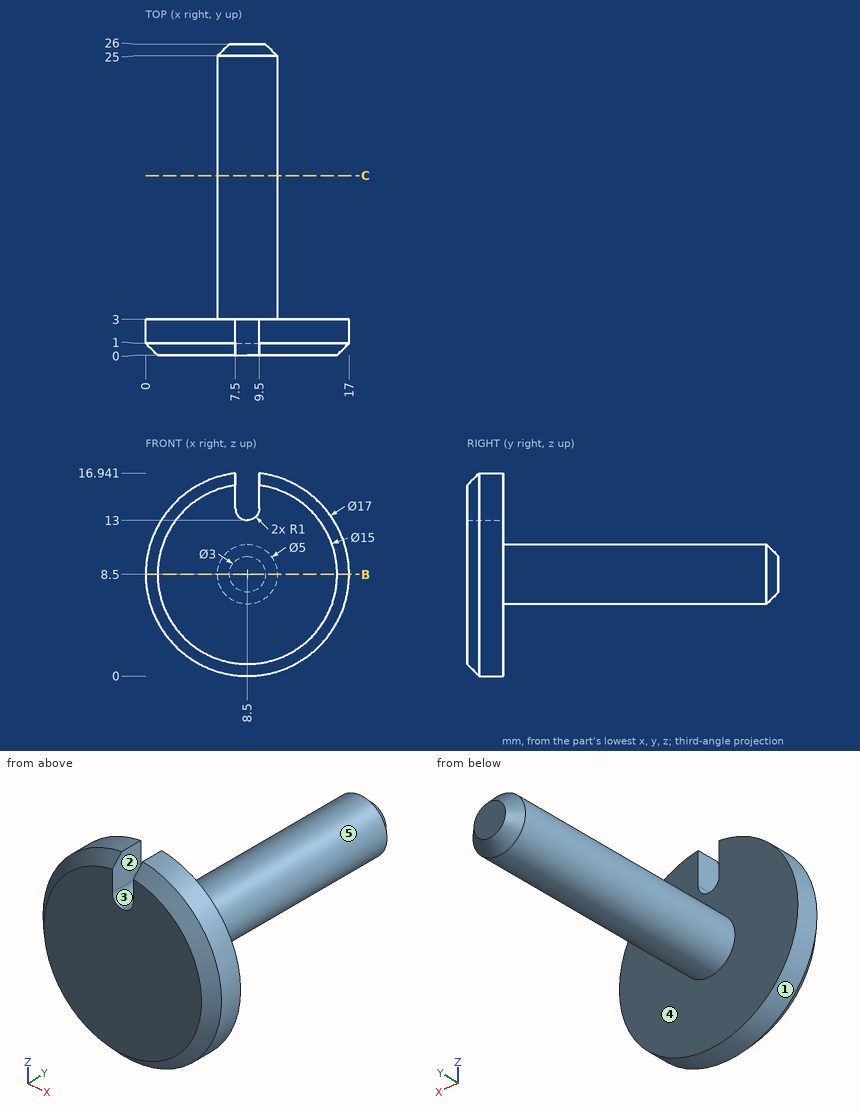
Job drawing, mm, ordinate dimensions from the low corner. One solid piece. A direction names the side the tool comes from. Give positions to 0.01 mm unless a question says otherwise; leave off trailing zeros. Loops run counter-clockwise (first coordinate to the right, second up) from the corner with the lowest first, then second, coordinate; pieces in that order, holes last. Notation, with made-up numbers: (10, -1.5) -> (32, -1.5) arc R9 ccw to (32, 10.5) -> close; hole circle Ø4 at (27.25, 68.25). An arc over 180 degrees is marked (long way). Write each question's results on one line, items separated by ' | '.
(1) Flat gauge pins, fed straight in: pin 1 Ø1 at (x, z) = (5, 8.5) entering from +Y; pin 2 Ø5 at (x, z) = (7, 13.5) entering from -Y; pin 3 Ø8 at (x, y) = (3, 7.5) entering from -Z; pin 4 Ø2.5 at (y, z) = (2, 15) entering from -X (3 decimals). Where does each tip first touch, or does it go through?
Geometry results:
pin 1: stops at y = 3 | pin 2: stops at y = 0 | pin 3: stops at z = 6.5 | pin 4: stops at x = 1.815
(2) Tool access for the marked faces 1 and 2: list every direction of +Z, -Z, +X, -X, +Y, -Y with a clear straight run to the whole face (end or side of a thin tool).
Geometry results:
face 1: +Y, -Y | face 2: +Z, +Y, -Y
(3) Probe line 1 along Y through (x, z) = (14, 8); line 2 along Z through (x, y) = (10.5, 9). List the from-to ranges inside material, lowest first.
Geometry results:
line 1: y = 0 to 3 | line 2: z = 7 to 10
(4) Cut at B-B on z = 8.5. List the corners of the cut face in (x, y), and give its area (3 significant figures).
Geometry results:
outline: (0, 1) -> (1, 0) -> (16, 0) -> (17, 1) -> (17, 3) -> (11, 3) -> (11, 25) -> (10, 26) -> (7, 26) -> (6, 25) -> (6, 3) -> (0, 3) -> close | area: 164 mm²
(5) Cut at C-C on y = 15. List the corners of the cut face in (x, z), and give its area (3 significant figures).
Geometry results:
outline: circle Ø5 at (8.5, 8.5) | area: 19.6 mm²
(6) Pull direction X, two halves, no side cores. Call the marked faces 3, 4 and 5: released by +X, released by -X, zero draft, split by the parting line, or undercut.
Geometry results:
face 3: undercut | face 4: zero draft | face 5: split by the parting line
